Design review of the part built by this model. Coordinates are the model's own, in mm. A direction names the side the tool comes from. Give positions to 0.01 mm unless a question says otherwise; leave off trailing zeros. Loops run counter-clockwise (first coordinate to the right, second up) from the corner with the lowest first, then second, coordinate; pieces in that order, holes last. Notation, with made-up numbers: (50.25, 41) -> (100.25, 41) arc R30 ccw to (100.25, 74) -> close; hole circle Ø4 at (-5, -20.75). An arc over 180 degrees is marked (long way). Answer in a Markdown table with one row per item. Add a question column.
(1) Consider section A-A on x = 5.5. Write out the cut boundary in (y, z).
(2) Consider section C-C on z = 22. Write out the cut boundary in (x, y).
(3) Consider section D-D on y = 15.5. Write out the cut boundary in (x, z), then the cut area to 3 significant figures.
(4) For faces 4 (the flat face through (0, 10, 15)), 5 (the flat face through (0, 15, 20)), 6 (the flat face through (0, 0, 0)), list the 3-axis set-ups (+Z, -Z, +X, -X, +Y, -Y) from which the entire face can be reached by the end or side of a thin tool; tool diameter is ignored.
(5) Consider section B-B on y = 2. Write out the cut boundary in (x, z), then the cut area to 3 significant figures.
(6) For line 1 (Z direction, x = 12.5, y = -8.5); line 2 (Z direction, x = 8, y = -11.5); line 3 (X direction, y = 6, z = 28), list the stretches that pass through material, from the lowest coordinate up.
(7) For pin 1 (11 mm diameter, centred on x = -1, y = -17.5, fed in from +Z); pin 2 (8 mm diameter, centred on x = 19, z = 17.5, fed in from -Y); pin 3 (3 mm diameter, centred on y = -17.5, z = 17, fed in from +X); pin 4 (12 mm diameter, centred on x = 11, y = -1.5, fed in from +Z), all flat-tipped, find the tip position at first contact; note any pin that passes through.
(8) Draft analysis for pull direction Y (two halves, no side actions). For faces 1 (the flat face through (-7, 20, 11)), 2 (the flat face through (0, -15, 20)), 3 (the flat face through (-10, 0, 22)), state which applies: +Y half, -Y half, draft (parallel to the pull), parting line (faces both ways), or undercut.
from build123d import *

# Parameters (mm, degrees)
F0_W     = 60
F0_H     = 40
F1_DEPTH = 10
F2_W     = 20
F2_H     = 40
F3_DEPTH = 20
F4_W     = 20
F4_H     = 10
F5_DEPTH = 10
F6_W     = 20
F6_H     = 10
F7_DEPTH = 10


with BuildPart() as f1:
    # F0 (on Top) → F1 (new body)
    with BuildSketch(Plane.XY):
        Rectangle(F0_W, F0_H)
    extrude(amount=F1_DEPTH)

    # F2 (on face) → F3 (join)
    with BuildSketch(Plane.XY.offset(10)):
        with Locations((-20, 0)):
            Rectangle(F2_W, F2_H)
    extrude(amount=F3_DEPTH)

    # F4 (on face) → F5 (join)
    with BuildSketch(Plane.XY.offset(10)):
        with Locations((0, -15)):
            Rectangle(F4_W, F4_H)
    extrude(amount=F5_DEPTH)

    # F6 (on face) → F7 (join)
    with BuildSketch(Plane.XY.offset(10)):
        with Locations((0, 15)):
            Rectangle(F6_W, F6_H)
    extrude(amount=F7_DEPTH)


solid = f1.part
Values follow:
| question | item | result |
|---|---|---|
| 1 | outline | (-20, 0) -> (20, 0) -> (20, 20) -> (10, 20) -> (10, 10) -> (-10, 10) -> (-10, 20) -> (-20, 20) -> close |
| 2 | outline | (-30, -20) -> (-10, -20) -> (-10, 20) -> (-30, 20) -> close |
| 3 | outline | (-30, 0) -> (30, 0) -> (30, 10) -> (10, 10) -> (10, 20) -> (-10, 20) -> (-10, 30) -> (-30, 30) -> close |
| 3 | area | 1,200 mm2 |
| 4 | face 4 | +Z, +X |
| 4 | face 5 | +Z, +X, +Y, -Y |
| 4 | face 6 | -Z, +X, -X, +Y, -Y |
| 5 | outline | (-30, 0) -> (30, 0) -> (30, 10) -> (-10, 10) -> (-10, 30) -> (-30, 30) -> close |
| 5 | area | 1,000 mm2 |
| 6 | line 1 | 0 to 10 |
| 6 | line 2 | 0 to 20 |
| 6 | line 3 | -30 to -10 |
| 7 | pin 1 | z = 20 |
| 7 | pin 2 | through |
| 7 | pin 3 | x = 10 |
| 7 | pin 4 | z = 10 |
| 8 | face 1 | +Y half |
| 8 | face 2 | draft |
| 8 | face 3 | undercut |
